```python
from build123d import *

# Parameters (mm, degrees)
EXTRUDE_1487_DEPTH     = 13
EXTRUDE_START          = -0.8
SKETCH_8_R             = 15
EXTRUDE_1654_DEPTH     = 0.8
CUT_EXTRUDE_1920_REACH = 69.233
SKETCH_1784_R          = 3.5
CUT_EXTRUDE_2148_REACH = 66.097
SKETCH_2017_R          = 3.5
CUT_EXTRUDE_2773_REACH = 66.097
CUT_EXTRUDE_2851_REACH = 66.897
CUT_EXTRUDE_START      = -0.8
SKETCH_3_W             = 5
SKETCH_3_H             = 6.5
SKETCH_3_R             = 1.5
FILLET_3030_R          = 3
FILLET_3594_R          = 3
EXTRUDE_START_2        = 2.2
SKETCH_4254_W          = 2.5
SKETCH_4254_H          = 2.5
EXTRUDE_4621_DEPTH     = 10.8
EXTRUDE_START_3        = 2.5
SKETCH_5_W             = 5
SKETCH_5_H             = 1.75
SKETCH_5_H_2           = 6.5
SKETCH_5_R             = 1.5
EXTRUDE_4751_DEPTH     = 2.5
FILLET_1_R             = 2.5


with BuildPart() as part:
    # Sketch 348 → Extrude 1487 (new body)
    with BuildSketch(Plane.XY):
        with BuildLine():
            Line((-10.3, -25.9), (10.3, -25.9))
            ThreePointArc((10.3, -25.9), (21.330865787, -21.330865787), (25.9, -10.3))
            Line((25.9, -10.3), (25.9, -7))
            Line((25.9, -7), (29.5, -7))
            Line((29.5, -7), (29.5, 7))
            Line((29.5, 7), (25.9, 7))
            Line((25.9, 7), (25.9, 10.3))
            ThreePointArc((25.9, 10.3), (21.330865787, 21.330865787), (10.3, 25.9))
            Line((10.3, 25.9), (7, 25.9))
            Line((7, 25.9), (7, 29.5))
            Line((7, 29.5), (-7, 29.5))
            Line((-7, 29.5), (-7, 25.9))
            Line((-7, 25.9), (-10.3, 25.9))
            ThreePointArc((-10.3, 25.9), (-21.330865787, 21.330865787), (-25.9, 10.3))
            Line((-25.9, 10.3), (-25.9, 7))
            Line((-25.9, 7), (-29.5, 7))
            Line((-29.5, 7), (-29.5, -7))
            Line((-29.5, -7), (-25.9, -7))
            Line((-25.9, -7), (-25.9, -10.3))
            ThreePointArc((-25.9, -10.3), (-21.330865787, -21.330865787), (-10.3, -25.9))
        make_face()
        with BuildLine():
            Line((-10.3, -24.3), (10.3, -24.3))
            ThreePointArc((10.3, -24.3), (20.199494937, -20.199494937), (24.3, -10.3))
            Line((24.3, -10.3), (24.3, -5.4))
            Line((24.3, -5.4), (27.9, -5.4))
            Line((27.9, -5.4), (27.9, 5.4))
            Line((27.9, 5.4), (24.3, 5.4))
            Line((24.3, 5.4), (24.3, 10.3))
            ThreePointArc((24.3, 10.3), (20.199494937, 20.199494937), (10.3, 24.3))
            Line((10.3, 24.3), (5.4, 24.3))
            Line((5.4, 24.3), (5.4, 27.9))
            Line((5.4, 27.9), (-5.4, 27.9))
            Line((-5.4, 27.9), (-5.4, 24.3))
            Line((-5.4, 24.3), (-10.3, 24.3))
            ThreePointArc((-10.3, 24.3), (-20.199494937, 20.199494937), (-24.3, 10.3))
            Line((-24.3, 10.3), (-24.3, 5.4))
            Line((-24.3, 5.4), (-27.9, 5.4))
            Line((-27.9, 5.4), (-27.9, -5.4))
            Line((-27.9, -5.4), (-24.3, -5.4))
            Line((-24.3, -5.4), (-24.3, -10.3))
            ThreePointArc((-24.3, -10.3), (-20.199494937, -20.199494937), (-10.3, -24.3))
        make_face(mode=Mode.SUBTRACT)
    extrude(amount=EXTRUDE_1487_DEPTH)

    # Эскиз-База<8> → Extrude 1654 (add)
    with BuildSketch(Plane.XY.offset(EXTRUDE_START)):
        with BuildLine():
            Line((-25.9, 7), (-29.5, 7))
            Line((-29.5, 7), (-29.5, -7))
            Line((-29.5, -7), (-25.9, -7))
            Line((-25.9, -7), (-25.9, -10.3))
            ThreePointArc((-25.9, -10.3), (-21.330865787, -21.330865787), (-10.3, -25.9))
            Line((-10.3, -25.9), (10.3, -25.9))
            ThreePointArc((10.3, -25.9), (21.330865787, -21.330865787), (25.9, -10.3))
            Line((25.9, -10.3), (25.9, -7))
            Line((25.9, -7), (29.5, -7))
            Line((29.5, -7), (29.5, 7))
            Line((29.5, 7), (25.9, 7))
            Line((25.9, 7), (25.9, 10.3))
            ThreePointArc((25.9, 10.3), (21.330865787, 21.330865787), (10.3, 25.9))
            Line((10.3, 25.9), (7, 25.9))
            Line((7, 25.9), (7, 29.5))
            Line((7, 29.5), (-7, 29.5))
            Line((-7, 29.5), (-7, 25.9))
            Line((-7, 25.9), (-10.3, 25.9))
            ThreePointArc((-10.3, 25.9), (-21.330865787, 21.330865787), (-25.9, 10.3))
            Line((-25.9, 10.3), (-25.9, 7))
        make_face()
        Circle(SKETCH_8_R, mode=Mode.SUBTRACT)
    extrude(amount=EXTRUDE_1654_DEPTH)

    # Sketch 1784 → Cut-Extrude 1920 (cut, up to next)
    with BuildSketch(Plane.ZY.offset(29.5), mode=Mode.PRIVATE) as cut_extrude_1920_sk1:
        with Locations(Location((6.1, 0, 0), (0, 0, 270))):
            Circle(SKETCH_1784_R)
    cut_extrude_1920_tool1 = extrude(cut_extrude_1920_sk1.sketch, amount=-CUT_EXTRUDE_1920_REACH, mode=Mode.PRIVATE) & part.part
    add(cut_extrude_1920_tool1.solids().sort_by_distance((-29.5, 0, 6.1))[0], mode=Mode.SUBTRACT)
    add(cut_extrude_1920_tool1.solids().sort_by_distance((-29.5, 0, 6.1))[1], mode=Mode.SUBTRACT)

    # Sketch 2017 → Cut-Extrude 2148 (cut, up to next)
    with BuildSketch(Plane(origin=(0, 29.5, 0), x_dir=(1, 0, 0), z_dir=(0, 1, 0)), mode=Mode.PRIVATE) as cut_extrude_2148_sk1:
        with Locations(Location((0, -6.1, 0), (0, 0, 180))):
            Circle(SKETCH_2017_R)
    cut_extrude_2148_tool1 = extrude(cut_extrude_2148_sk1.sketch, amount=-CUT_EXTRUDE_2148_REACH, mode=Mode.PRIVATE) & part.part
    add(cut_extrude_2148_tool1.solids().sort_by_distance((0, 29.5, 6.1))[0], mode=Mode.SUBTRACT)

    # Sketch 2270 → Cut-Extrude 2773 (cut, up to next)
    with BuildSketch(Plane.XZ.offset(25.9), mode=Mode.PRIVATE) as cut_extrude_2773_sk1:
        Polygon((3.5, 11.5), (3.5, 4), (2.5, 4), (2.5, 10.5), (-2.5, 10.5), (-2.5, 4), (-3.5, 4), (-3.5, 11.5), align=None)
    cut_extrude_2773_tool1 = extrude(cut_extrude_2773_sk1.sketch, amount=-CUT_EXTRUDE_2773_REACH, mode=Mode.PRIVATE) & part.part
    add(cut_extrude_2773_tool1.solids().sort_by_distance((3.397409, -25.9, 7.75))[0], mode=Mode.SUBTRACT)

    # Эскиз-Кнопка записи<3> → Cut-Extrude 2851 (cut, up to next)
    with BuildSketch(Plane.XZ.offset(25.9).offset(CUT_EXTRUDE_START), mode=Mode.PRIVATE) as cut_extrude_2851_sk1:
        with Locations((0, 7.25)):
            Rectangle(SKETCH_3_W, SKETCH_3_H)
        with Locations(Location((0, 7.75, 0), (0, 0, 270))):
            Circle(SKETCH_3_R, mode=Mode.SUBTRACT)
    cut_extrude_2851_tool1 = extrude(cut_extrude_2851_sk1.sketch, amount=-CUT_EXTRUDE_2851_REACH, mode=Mode.PRIVATE) & part.part
    add(cut_extrude_2851_tool1.solids().sort_by_distance((-2.417994, -25.1, 7.25))[0], mode=Mode.SUBTRACT)

    # Fillet 3030
    fillet_3030_edges = [part.edges().sort_by_distance(p)[0] for p in [
        (-7.85, 24.3, 0),
        (-20.199494937, 20.199494937, 0),
        (-24.3, -7.85, 0),
        (-20.199494937, -20.199494937, 0),
        (20.199494937, -20.199494937, 0),
        (20.199494937, 20.199494937, 0),
        (7.85, 24.3, 0),
        (24.3, 7.85, 0),
        (24.3, -7.85, 0),
        (0, -24.3, 0),
        (-24.3, 7.85, 0),
    ]]
    fillet(fillet_3030_edges, radius=FILLET_3030_R)

    # Fillet 3594
    fillet_3594_edges = [part.edges().sort_by_distance(p)[0] for p in [
        (-21.330865787, 21.330865787, -0.8),
        (-8.65, 25.9, -0.8),
        (8.65, 25.9, -0.8),
        (21.330865787, 21.330865787, -0.8),
        (25.9, 8.65, -0.8),
        (25.9, -8.65, -0.8),
        (21.330865787, -21.330865787, -0.8),
        (0, -25.9, -0.8),
        (-21.330865787, -21.330865787, -0.8),
        (-25.9, -8.65, -0.8),
        (-25.9, 8.65, -0.8),
    ]]
    fillet(fillet_3594_edges, radius=FILLET_3594_R)

    # Sketch 4254 → Extrude 4621 (add)
    with BuildSketch(Plane.XY.offset(EXTRUDE_START_2)):
        Polygon((-9.5, 25.9), (-9.5, 28.4), (-12.5, 28.4), (-12.5, 25.4), align=None)
        Polygon((12, -25.4), (9.5, -25.9), (9.5, -28.4), (12, -28.4), align=None)
        Polygon((9.5, 25.9), (9.5, 28.4), (12.5, 28.4), (12.5, 25.4), align=None)
        Polygon((-9.5, -25.9), (-9.5, -28.4), (-12, -28.4), (-12, -25.4), align=None)
        with Locations((-5.75, -27.15)):
            Rectangle(SKETCH_4254_W, SKETCH_4254_H)
        with Locations((5.75, -27.15)):
            Rectangle(SKETCH_4254_W, SKETCH_4254_H)
    extrude(amount=EXTRUDE_4621_DEPTH)

    # Эскиз-Кнопка записи<5> → Extrude 4751 (add)
    # profile 1 of 3: a face of its own
    with BuildSketch(Plane.XZ.offset(25.9).offset(EXTRUDE_START_3)):
        with Locations((0, 3.125)):
            Rectangle(SKETCH_5_W, SKETCH_5_H)
    # profile 2 of 3: a face of its own
    with BuildSketch(Plane.XZ.offset(25.9).offset(EXTRUDE_START_3)):
        with Locations((0, 7.25)):
            Rectangle(SKETCH_5_W, SKETCH_5_H_2)
        with Locations(Location((0, 7.75, 0), (0, 0, 270))):
            Circle(SKETCH_5_R, mode=Mode.SUBTRACT)
    # profile 3 of 3: a face of its own
    with BuildSketch(Plane.XZ.offset(25.9).offset(EXTRUDE_START_3)):
        with Locations(Location((0, 7.75, 0), (0, 0, 270))):
            Circle(SKETCH_5_R)
    extrude(amount=-EXTRUDE_4751_DEPTH)

    # Скругление1
    fillet_1_edges = [part.edges().sort_by_distance(p)[0] for p in [
        (10.75, -28.4, 2.2),
        (5.75, -28.4, 2.2),
        (-10.75, -28.4, 2.2),
        (-5.75, -28.4, 2.2),
        (0, -28.4, 2.25),
        (11, 28.4, 2.2),
        (-11, 28.4, 2.2),
    ]]
    fillet(fillet_1_edges, radius=FILLET_1_R - 0.0001)  # a hair under: the kernel refuses the full size


solid = part.part
```
Check sheet for the modelled part. Datum: model origin and axes. Units: mm. A direction names the side the tool comes from. Give positions to 0.01 mm unless a question says otherwise; leave off trailing zeros. Loops run counter-clockwise (first coordinate to the right, second up) from the corner with the lowest first, then second, coordinate; pieces in that order, holes last. Notation, with made-up numbers: (41.25, 89.25) - (86.25, 89.25) arc R19 cw to (86.25, 119.25) - close; hole circle Ø4 at (8.25, 69.25). An arc over 180 degrees is marked (long way). One line per question, with ' | ' between items. Start each with the question number.
1. Cross-section at A-A, the plane y = 2. Enter the section's corners in (x, z).
2. Gauge pin test, flat ends, axial feed: pin 1 Ø5 at (y, z) = (-17.5, 5.5) entering from +X; pin 2 Ø7.5 at (x, z) = (25.5, 4.5) entering from -Y; pin 3 Ø1.3 at (y, z) = (-27.5, 5.5) entering from +X; pin 4 Ø5.5 at (y, z) = (0, 6.1) entering from +X. Record the tip position at first contact, or that the pin passes through.
3. Cross-section at B-B, the plane z = 8.25. Give the number of separate pieces and of enclosed holes in the cut face, plus the area to 3 significant figures.
4. Draft check along Y on faces 4 (the flat face through (-11, -28.4, 9)), 5 (the cylindrical face through (-20.1, 20.3, 7.9)), 6 (the cylindrical face through (0.759, 28.711, 2.683)). Enter one of: released by +Y, released by -Y, zero draft, split by the parting line, or undercut.
5. Set-up check for faces 1 (the flat face through (25.9, -9, 8)), 2 (the cylindrical face through (0.14, -23.4, 0.86)), 3 (the cylindrical face through (-25, -8.67, 0.06)): record each of +Z, -Z, +X, -X, +Y, -Y from which the full face is reachable in a straight line by a thin tool's end or side.
6. Material ranges on line 1 along Z through (x, y) = (28, 0); line 2 along X through (y, z) = (10, 10.75); line 3 along Y through (x, z) = (-3, 3.25), recorded low to high. Write a range as [from, to].
Check result:
1) outline: (-29.5, -0.8) - (-14.87, -0.8) - (-14.87, 0) - (-27.9, 0) - (-27.9, 3.23) - (-29.5, 3.23) - close; (-29.5, 8.97) - (-27.9, 8.97) - (-27.9, 13) - (-29.5, 13) - close; (14.87, -0.8) - (29.5, -0.8) - (29.5, 3.23) - (27.9, 3.23) - (27.9, 0) - (14.87, 0) - close; (27.9, 8.97) - (29.5, 8.97) - (29.5, 13) - (27.9, 13) - close
2) pin 1: stops at x = 25.18 | pin 2: stops at y = -20.9 | pin 3: stops at x = 12 | pin 4: passes through
3) separate pieces: 5 | enclosed holes: 0 | area: 337 mm2
4) face 4: released by -Y | face 5: undercut | face 6: zero draft
5) face 1: +Z, -Z, +X, -Y | face 2: +Z | face 3: -Z, -X, -Y
6) line 1: z = [-0.8, 2.6], [9.6, 13] | line 2: x = [-25.9, -24.3], [24.3, 25.9] | line 3: y = [-25.9, -24.3], [27.9, 29.5]
